The figure shows three views and two pictorial views of one solid part (mm, origin at its lowest corner). Answer the questions. A direction names the side the tool comes from. Give positions to 0.01 mm unless a question says otherwise; leave off trailing zeros. Write each loop counter-clockwise with the first axis right and the second up, starting at its lowest first coordinate (ties: lowest second). Pieces come first, ordered by that corner, then holes. Notation, with made-up numbers: (13.5, -12) - (67.5, -12) arc R8 ccw to (67.5, -2) - close; hole circle Ø3 at (78.25, 63). An arc over 180 degrees is marked (long way). Write each question's results on one line, items separated by ' | '. Start each with the question number.
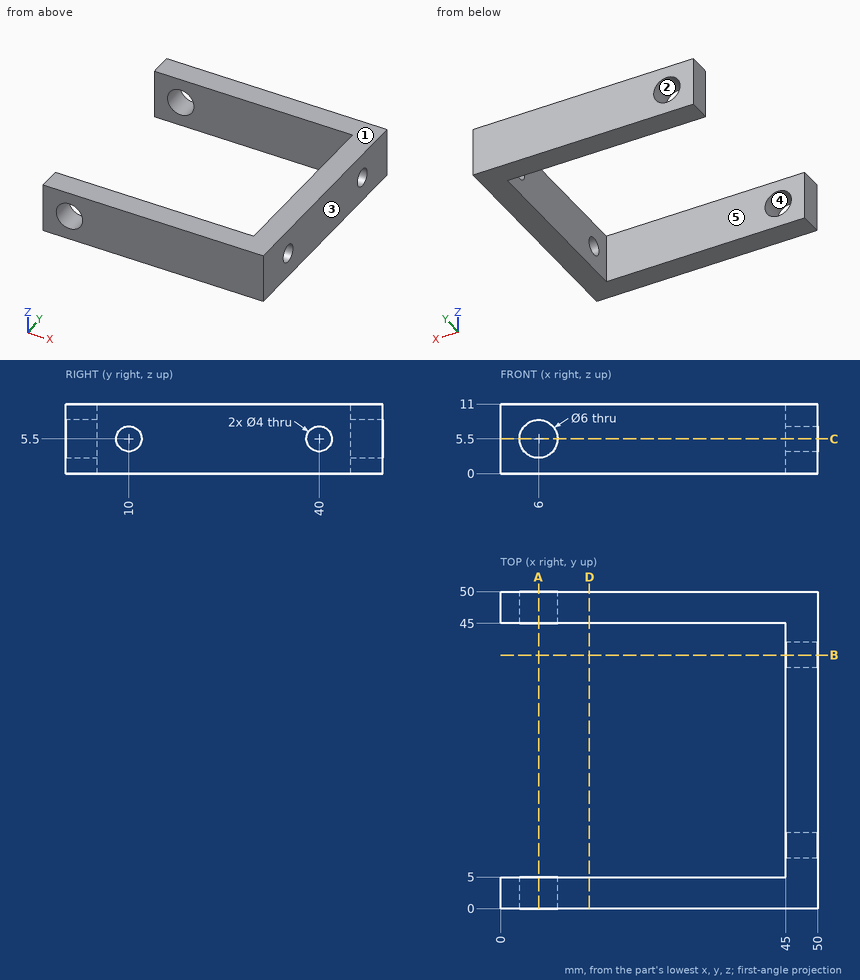
Q1. A tool of negligible diameter and unlimited length cuts with its end or side. For the marked faces 4 and 5, from which of +Z, -Z, +X, -X, +Y, -Y can it reach the whole face along a straight path? Write none if from no direction.
Q2. A cutting plane is placed at A-A, the plane x = 6. Write down the section's boundary in (y, z), and give its area (3 significant figures).
Q3. A cutting plane is placed at C-C, the plane z = 5.5. Write down the section's boundary in (x, y).
Q4. A cutting plane is placed at D-D, the plane x = 14. Write down the section's boundary in (y, z), and give its area (3 significant figures).
Q5. A cutting plane is placed at B-B, the plane y = 40. Write down the section's boundary in (x, z), and give its area (3 significant figures).
Q6. The mould has two halves that part along Z. Classify the marked faces 1, 2 and 3: pulls with the +Z half, pulls with the -Z half, needs draft (parallel to the pull), parting line crosses it, or undercut.
Q7. Consider L1, parallel to Y at x = 48.85, z = 5.5; L2, parallel to Y at x = 13, z = 2.75; L3, parallel to X at y = 2.25, z = 5.5. Determine where each line is inside the solid, lowest interval first.
Result:
1) face 4: +Y, -Y | face 5: +Z, -Z, -X
2) outline: (0, 0) - (5, 0) - (5, 2.5) - (0, 2.5) - close; (0, 8.5) - (5, 8.5) - (5, 11) - (0, 11) - close; (45, 0) - (50, 0) - (50, 2.5) - (45, 2.5) - close; (45, 8.5) - (50, 8.5) - (50, 11) - (45, 11) - close | area: 50.0 mm2
3) outline: (0, 0) - (3, 0) - (3, 5) - (0, 5) - close; (0, 45) - (3, 45) - (3, 50) - (0, 50) - close; (9, 0) - (50, 0) - (50, 8) - (45, 8) - (45, 5) - (9, 5) - close; (9, 45) - (45, 45) - (45, 42) - (50, 42) - (50, 50) - (9, 50) - close; (45, 12) - (50, 12) - (50, 38) - (45, 38) - close
4) outline: (0, 0) - (5, 0) - (5, 11) - (0, 11) - close; (45, 0) - (50, 0) - (50, 11) - (45, 11) - close | area: 110 mm2
5) outline: (45, 0) - (50, 0) - (50, 3.5) - (45, 3.5) - close; (45, 7.5) - (50, 7.5) - (50, 11) - (45, 11) - close | area: 35.0 mm2
6) face 1: pulls with the +Z half | face 2: undercut | face 3: needs draft
7) L1: y = 0 to 8, 12 to 38, 42 to 50 | L2: y = 0 to 5, 45 to 50 | L3: x = 0 to 3, 9 to 50
